Here's how the part is built. I have some questions about the finished solid (model axes, mm). Face numbers are marked on the shaded views. A direction names the side the tool comes from. Coordinates: 2 decimals unless noted, no trailing zeros. Write each loop counter-clockwise with the first axis right and the second up, starting at its lowest first coordinate (ties: lowest second). Pieces come first, ordered by that corner, then holes.
Item 1: If we section it at B-B (z = -5.5): Please give me the cut outline in (x, y) (3 decimals).
Item 2: If we section it at D-D (y = -3): Please give me the cut outline in (x, z).
Item 3: We'd pull the mould along Z, two halves only. Please class the marked faces 4, 5 and 6: +Z half, -Z half, draft (parallel to the pull), parting line (faces both ways), or undercut.
Item 4: I'm going to push flat-ended pins straight in: pin 1 Ø0.8 at (x, z) = (2.5, 3) entering from +Y; pin 2 Ø2 at (x, y) = (2.5, -8.5) entering from +Z; pin 3 Ø1.8 at (x, z) = (0, 1) entering from +Y (3 decimals). Where does each tip first touch, or does it pass through?
Item 5: For the marked faces 1, 2 and 3, which set-ups out of +Z, -Z, +X, -X, +Y, -Y let a thin tool reach every point of the face, with its end or its side?
Item 6: If we section it at C-C (z = -12.5): Please give me the cut outline in (x, y), then the cut area to 3 significant figures.
Item 7: If we section it at A-A (x = 0): Please give me the cut outline in (y, z) (3 decimals), then the cut area to 3 significant figures.
Item 8: If I drill on line 1 (Z direction, x = 0, y = -0.35); line 2 (Z direction, x = -1, y = -3.5); line 3 (Z direction, x = 0, y = -8), over which ranges is the centre line in solid material (lowest first)?
from build123d import *

# Parameters (mm, degrees)
F0_R           = 3.75
F0_R_2         = 2.55
F0_R_3         = 2.45
F1_DEPTH       = 4.9
F6_R           = 2.45
F7_DEPTH       = 5
F8_D           = 2.8
F8_CBORE_D     = 3.8
F8_CBORE_DEPTH = 1.5


with BuildPart() as f1:
    # F0 (on Front) → F1 (new body)
    with BuildSketch(Plane.XZ):
        with Locations((0, -10.556)):
            Circle(F0_R)
        with Locations((0, -10.556)):
            Circle(F0_R_2, mode=Mode.SUBTRACT)
        with Locations((0, 10.556)):
            Circle(F0_R)
        with Locations((0, 10.556)):
            Circle(F0_R_3, mode=Mode.SUBTRACT)
        with Locations((0, 10.556)):
            Circle(F0_R_3)
    extrude(amount=F1_DEPTH)

    # F2 (on Top) → F3 (join, up to the next surface of F1)
    with BuildSketch(Plane.XY):
        with BuildLine():
            Line((-2, -0.45), (-2.75, -0.45))
            ThreePointArc((-2.75, -0.45), (-3.1035533906, -0.5964466094), (-3.25, -0.95))
            Line((-3.25, -0.95), (-3.25, -3.95))
            ThreePointArc((-3.25, -3.95), (-3.1035533906, -4.3035533906), (-2.75, -4.45))
            Line((-2.75, -4.45), (-2, -4.45))
            ThreePointArc((-2, -4.45), (-1.8232233047, -4.3767766953), (-1.75, -4.2))
            Line((-1.75, -4.2), (-1.75, -4.075))
            Line((-1.75, -4.075), (1.75, -4.075))
            Line((1.75, -4.075), (1.75, -4.2))
            ThreePointArc((1.75, -4.2), (1.8232233047, -4.3767766953), (2, -4.45))
            Line((2, -4.45), (2.75, -4.45))
            ThreePointArc((2.75, -4.45), (3.1035533906, -4.3035533906), (3.25, -3.95))
            Line((3.25, -3.95), (3.25, -0.95))
            ThreePointArc((3.25, -0.95), (3.1035533906, -0.5964466094), (2.75, -0.45))
            Line((2.75, -0.45), (2, -0.45))
            ThreePointArc((2, -0.45), (1.8232233047, -0.5232233047), (1.75, -0.7))
            Line((1.75, -0.7), (1.75, -0.825))
            Line((1.75, -0.825), (-1.75, -0.825))
            Line((-1.75, -0.825), (-1.75, -0.7))
            ThreePointArc((-1.75, -0.7), (-1.8232233047, -0.5232233047), (-2, -0.45))
        make_face()
    extrude(until=Until.NEXT)

    # F3_face (on face) → F4 (join, up to the next surface of F1)
    with BuildSketch(Plane(origin=(0, -2.45, 0), x_dir=(1, 0, 0), z_dir=(0, 0, -1))):
        with BuildLine():
            Line((2, -2), (2.75, -2))
            ThreePointArc((2.75, -2), (3.1035533906, -1.8535533906), (3.25, -1.5))
            Line((3.25, -1.5), (3.25, 1.5))
            ThreePointArc((3.25, 1.5), (3.1035533906, 1.8535533906), (2.75, 2))
            Line((2.75, 2), (2, 2))
            ThreePointArc((2, 2), (1.8232233047, 1.9267766953), (1.75, 1.75))
            Line((1.75, 1.75), (1.75, 1.625))
            Line((1.75, 1.625), (-1.75, 1.625))
            Line((-1.75, 1.625), (-1.75, 1.75))
            ThreePointArc((-1.75, 1.75), (-1.8232233047, 1.9267766953), (-2, 2))
            Line((-2, 2), (-2.75, 2))
            ThreePointArc((-2.75, 2), (-3.1035533906, 1.8535533906), (-3.25, 1.5))
            Line((-3.25, 1.5), (-3.25, -1.5))
            ThreePointArc((-3.25, -1.5), (-3.1035533906, -1.8535533906), (-2.75, -2))
            Line((-2.75, -2), (-2, -2))
            ThreePointArc((-2, -2), (-1.8232233047, -1.9267766953), (-1.75, -1.75))
            Line((-1.75, -1.75), (-1.75, -1.625))
            Line((-1.75, -1.625), (1.75, -1.625))
            Line((1.75, -1.625), (1.75, -1.75))
            ThreePointArc((1.75, -1.75), (1.8232233047, -1.9267766953), (2, -2))
        make_face()
    extrude(until=Until.NEXT)

    # F6 (on face) → F7 (join)
    with BuildSketch(Plane.XZ.offset(4.9)):
        with Locations((0, 10.556)):
            Circle(F6_R)
    extrude(amount=F7_DEPTH)

    # F8 (through all)
    with Locations(Plane(origin=(0, 0, 0), x_dir=(-1, 0, 0), z_dir=(0, 1, 0))):
        with Locations((0, 10.556)):
            CounterBoreHole(F8_D / 2, F8_CBORE_D / 2, F8_CBORE_DEPTH)


solid = f1.part
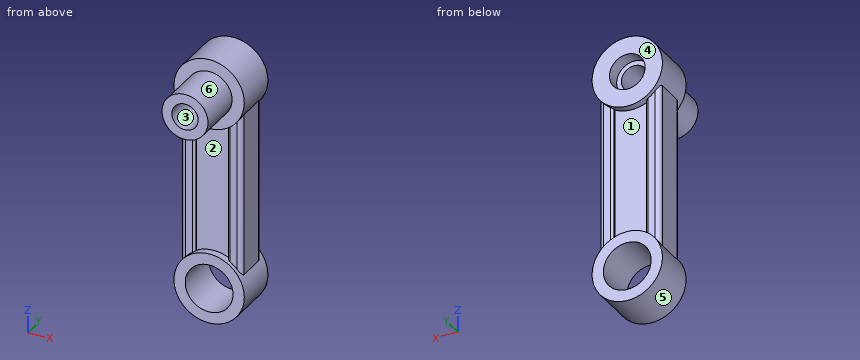
Answer list:
1. outline: (-3.25, -3.95) arc R0.5 ccw to (-2.75, -4.45) - (-2, -4.45) arc R0.25 ccw to (-1.75, -4.2) - (-1.75, -4.075) - (1.75, -4.075) - (1.75, -4.2) arc R0.25 ccw to (2, -4.45) - (2.75, -4.45) arc R0.5 ccw to (3.25, -3.95) - (3.25, -0.95) arc R0.5 ccw to (2.75, -0.45) - (2, -0.45) arc R0.25 ccw to (1.75, -0.7) - (1.75, -0.825) - (-1.75, -0.825) - (-1.75, -0.7) arc R0.25 ccw to (-2, -0.45) - (-2.75, -0.45) arc R0.5 ccw to (-3.25, -0.95) - close
2. outline: (-3.25, -8.69) arc R3.75 ccw (long way) to (3.25, -8.69) - (3.25, 8.69) arc R3.75 ccw (long way) to (-3.25, 8.69) - close; hole circle Ø5.1 at (0, -10.56); hole circle Ø2.8 at (0, 10.56)
3. face 4: draft
3. face 5: undercut
3. face 6: parting line
4. pin 1: stops at y = -0.45
4. pin 2: stops at z = 12.49
4. pin 3: stops at y = -0.825
5. face 1: +Y
5. face 2: -Y
5. face 3: +Y, -Y
6. outline: (-3.21, -4.9) - (-1.65, -4.9) - (-1.65, 0) - (-3.21, 0) - close; (1.65, -4.9) - (3.21, -4.9) - (3.21, 0) - (1.65, 0) - close
6. area: 15.3 mm2
7. outline: (-9.9, 8.106) - (-4.9, 8.106) - (-4.9, 6.806) - (-4.075, 6.806) - (-4.075, -6.806) - (-4.9, -6.806) - (-4.9, -8.006) - (0, -8.006) - (0, -6.806) - (-0.825, -6.806) - (-0.825, 6.806) - (0, 6.806) - (0, 8.656) - (-1.5, 8.656) - (-1.5, 9.156) - (-9.9, 9.156) - close; (-9.9, 11.956) - (-1.5, 11.956) - (-1.5, 12.456) - (0, 12.456) - (0, 14.306) - (-4.9, 14.306) - (-4.9, 13.006) - (-9.9, 13.006) - close; (-4.9, -14.306) - (0, -14.306) - (0, -13.106) - (-4.9, -13.106) - close
7. area: 88.0 mm2
8. line 1: z = -14.31 to -13.11, -8.01 to -6.81, 6.81 to 8.66, 12.46 to 14.31
8. line 2: z = -14.17 to -12.9, -8.21 to 9.58, 11.54 to 14.17
8. line 3: z = 8.11 to 9.16, 11.96 to 13.01
